Geometry: final body of the model. Coordinates: model frame, mm. A direction names the side the tool comes from. Give positions to 0.01 mm unless a question says otherwise; leave off trailing zeros. Order: outer loops, then holes, each group sorted by start corner. A loop starts at its lowest first (then second) coordinate and runs counter-clockwise, first axis right, second up. Notation, with made-up numbers: M -26.5,43 L -10.5,43 A24 cw -10.5,77 Z; hole C -35.5,-39 d10. An arc over 180 degrees is marked long. Use CSV: the item, a comma, the result in double quotes.
```python
from build123d import *

# Parameters (mm, degrees)
F0_R     = 22.225
F0_R_2   = 12.7
F1_DEPTH = 44.45
F3_DEPTH = 38.1
F4_R     = 6.35
F5_DEPTH = 12.7
F7_DEPTH = 6.35


with BuildPart() as f1:
    # F0 (on Front) → F1 (new body, symmetric)
    with BuildSketch(Plane.XZ):
        Circle(F0_R)
        Circle(F0_R_2, mode=Mode.SUBTRACT)
    extrude(amount=F1_DEPTH, both=True)

    # F2 (on Front) → F3 (join, symmetric)
    with BuildSketch(Plane.XZ):
        with BuildLine():
            ThreePointArc((0, -22.225), (-3.208614, -21.992167), (-6.35, -21.298547))
            Line((-6.35, -21.298547), (-6.35, -88.9))
            Line((-6.35, -88.9), (0, -88.9))
            Line((0, -88.9), (0, -22.225))
        make_face()
        with BuildLine():
            ThreePointArc((6.35, -21.298547), (3.208614, -21.992167), (0, -22.225))
            Line((0, -22.225), (0, -88.9))
            Line((0, -88.9), (6.35, -88.9))
            Line((6.35, -88.9), (6.35, -21.298547))
        make_face()
    extrude(amount=F3_DEPTH, both=True)

    # F4 (on face) → F5 (join)
    with BuildSketch(Plane(origin=(0, 0, -88.9), x_dir=(1, 0, 0), z_dir=(0, 0, -1))):
        with BuildLine():
            Line((6.35, -38.1), (6.35, 38.1))
            Line((6.35, 38.1), (-53.975, 38.1))
            ThreePointArc((-53.975, 38.1), (-65.20032, 33.45032), (-69.85, 22.225))
            Line((-69.85, 22.225), (-69.85, -22.225))
            ThreePointArc((-69.85, -22.225), (-65.20032, -33.45032), (-53.975, -38.1))
            Line((-53.975, -38.1), (6.35, -38.1))
        make_face()
        with Locations((-53.975, -22.225)):
            Circle(F4_R, mode=Mode.SUBTRACT)
        with Locations((-22.225, -22.225)):
            Circle(F4_R, mode=Mode.SUBTRACT)
        with Locations((-53.975, 22.225)):
            Circle(F4_R, mode=Mode.SUBTRACT)
        with Locations((-22.225, 22.225)):
            Circle(F4_R, mode=Mode.SUBTRACT)
    extrude(amount=-F5_DEPTH)

    # F6 (on Front) → F7 (join, symmetric)
    with BuildSketch(Plane.XZ):
        with BuildLine():
            ThreePointArc((-6.35, -21.298547), (-20.656868, -8.200269), (-19.229016, 11.144306))
            Line((-19.229016, 11.144306), (-69.85, -76.2))
            Line((-69.85, -76.2), (-53.975, -76.2))
            Line((-53.975, -76.2), (-6.35, -76.2))
            Line((-6.35, -76.2), (-6.35, -21.298547))
        make_face()
    extrude(amount=F7_DEPTH, both=True)


solid = f1.part
```
1. Line query: line 1 (Z direction, x = 0, y = 6) (3 decimals); line 2 (X direction, y = 26.5, z = -69); line 3 (Z direction, x = 7.5, y = 0.5). Output: solid intervals per line, ascending.
Answer:
line 1,"-88.9 to -12.7, 12.7 to 22.225"
line 2,"-6.35 to 6.35"
line 3,"-20.92 to -10.25, 10.25 to 20.92"
2. Section C-C, the plane z = -7. Return the cut outline in (x, y).
Answer:
outline,"M -29.74,-6.35 L -21.09,-6.35 L -21.09,-44.45 L -10.6,-44.45 L -10.6,44.45 L -21.09,44.45 L -21.09,6.35 L -29.74,6.35 Z; M 10.6,-44.45 L 21.09,-44.45 L 21.09,44.45 L 10.6,44.45 Z"
3. Reachability of faces 1 (the face through (-39, 22, -76.2)), 2 (the face through (-26.905, 17.933, -82.639)), 3 (the face through (11.95, -0.62, 18.74)), 4 (the face through (-6.35, -22, -48)), 5 (the face through (6.35, -1, -56)) from +Z, -Z, +X, -X, +Y, -Y: full face, straight path, thin tool, end or side. Return the list, or none.
Answer:
face 1,"-X, +Y"
face 2,"-Z"
face 3,"none"
face 4,"-X, -Y"
face 5,"-Z, +X, +Y, -Y"
4. Section A-A, the plane x = 0. Return the cut outline in (y, z) (3 decimals), plus the area to 3 significant figures.
Answer:
outline,"M -44.45,-22.225 L -38.1,-22.225 L -38.1,-88.9 L 38.1,-88.9 L 38.1,-22.225 L 44.45,-22.225 L 44.45,-12.7 L -44.45,-12.7 Z; M -44.45,12.7 L 44.45,12.7 L 44.45,22.225 L -44.45,22.225 Z"
area,"6,770 mm2"
5. Pull-direction query (Z, two-part tool) for faces 6 (the face through (-31, 6.35, -51)), 7 (the face through (-32, -1, -88.9)), 8 (the face through (-4, 38.1, -70)), 9 (the face through (-2.75, 0.62, -12.4)); classes: +Z half, -Z half, draft (parallel to the pull), parting line (faces both ways), or undercut.
Answer:
face 6,"undercut"
face 7,"-Z half"
face 8,"draft"
face 9,"undercut"
6. Pin query (flat end, axial travel): pin 1 Ø7.5 at (x, y) = (-22.225, -22.225) entering from -Z; pin 2 Ø20.5 at (x, y) = (-53.975, -22.225) entering from +Z; pin 3 Ø2 at (x, z) = (-1.5, -56) entering from -Y; pin 4 Ø15 at (x, z) = (0, 0) entering from +Y. Return the tip coordinate at first contact, or that it passes through.
Answer:
pin 1,"z = -12.35"
pin 2,"z = -76.2"
pin 3,"y = -38.1"
pin 4,"through"
7. Section D-D, the plane y = 20. Return the cut outline in (x, z) (3 decimals), plus the area to 3 significant figures.
Answer:
outline,"M -69.85,-88.9 L -59.922,-88.9 L -59.922,-76.2 L -69.85,-76.2 Z; M -48.028,-88.9 L -28.172,-88.9 L -28.172,-76.2 L -48.028,-76.2 Z; M -16.278,-88.9 L 6.35,-88.9 L 6.35,-21.299 A22.225 ccw long -6.35,-21.299 L -6.35,-76.2 L -16.278,-76.2 Z; hole C 0,0 d25.4"
area,"2,400 mm2"
8. Section B-B, the plane y = 11. Return the cut outline in (x, z) (3 decimals), plus the area to 3 significant figures.
Answer:
outline,"M -69.85,-88.9 L 6.35,-88.9 L 6.35,-21.299 A22.225 ccw long -6.35,-21.299 L -6.35,-76.2 L -69.85,-76.2 Z; hole C 0,0 d25.4"
area,"2,700 mm2"
